```python
from build123d import *

# Parameters (mm, degrees)
SKETCH1_W       = 3
SKETCH1_H       = 12
SKETCH5_W       = 2.05
SKETCH5_H       = 0.74
CHANFREIN1_SIZE = 0.2


with BuildPart() as part:
    # Sketch1 → Revolve1 (revolve)
    with BuildSketch(Plane.XY):
        with Locations((1.5, 6)):
            Rectangle(SKETCH1_W, SKETCH1_H)
    revolve(axis=Axis((0, 0, 0), (0, 1, 0)))

    # Sketch5 → Groove for DIN 471 - 4 x 0.4, Circlip for shafts - normal1 (revolve, cut)
    with BuildSketch(Plane(origin=(0, 0, 0), x_dir=(0, 0, -1), z_dir=(-1, 0, 0))):
        with Locations((3.525, -10.97)):
            Rectangle(SKETCH5_W, SKETCH5_H)
    revolve(axis=Axis((0, 50.028808754, 0), (0, -1, 0)), mode=Mode.SUBTRACT)

    # Chanfrein1
    chanfrein1_edges = [part.edges().sort_by_distance(p)[0] for p in [
        (-3, 0, 0),
        (-3, 12, 0),
    ]]
    chamfer(chanfrein1_edges, length=CHANFREIN1_SIZE)


solid = part.part
```
Verification items for the finished model (mm, model axes). A direction names the side the tool comes from. Round coordinates to 2 decimals unless told otherwise and drop trailing zeros. Write each loop counter-clockwise with the first axis right and the second up, starting at its lowest first coordinate (ties: lowest second). Pieces come first, ordered by that corner, then holes. Notation, with made-up numbers: (84.25, 48.5) - (111.25, 48.5) arc R20 cw to (111.25, 63.5) - close; hole circle Ø4 at (68, 70). An arc over 180 degrees is marked (long way). Answer as a JSON object with one key per item and string values. Group by question number.
Q1. Section check A-A, the plane y = 11. Enter the section's corners in (x, z).
Q2. Section check B-B, the plane y = 5. Enter the section's corners in (x, z), plus the area to 3 significant figures.
Q3. Thickness scan on line 1 (Y direction, x = 0.9, z = -2.55); line 2 (Z direction, x = -1.7, y = 8.75); line 3 (Z direction, x = -1, y = 8.75). Record the ranges inside material, lowest first.
Q4. Go/stop test with a flat-tipped pin: pin 1 Ø3 at (x, y) = (2, 10.5) entering from -Z. Record where the tip stops, or that it passes through.
Q5. Tool access check on faces 1 (the cylindrical face through (-2.44, 10.96, 0.54)), 2 (the cylindrical face through (-3, 11.6, -0.1)). Record the directions out of +Z, -Z, +X, -X, +Y, -Y that give a thin tool (end or side, any length) a straight path to the whole face; none if there is none.
Q6. Mould release check, pull along Y, two halves, no side actions. Record for faces 3 (the flat face through (2, 11.34, -2)), 4 (the flat face through (0, 0, 0)), 5 (the flat face through (0, 12, 0)): released by +Y, released by -Y, zero draft, split by the parting line, or undercut.
Found:
{
 "1": {"outline": "circle Ø5 at (0, 0)"},
 "2": {"outline": "circle Ø6 at (0, 0)", "area": "28.3 mm^2"},
 "3": {"line 1": "y = 0 to 10.6, 11.34 to 12", "line 2": "z = -2.47 to 2.47", "line 3": "z = -2.83 to 2.83"},
 "4": {"pin 1": "stops at z = -2.96"},
 "5": {"face 1": "none", "face 2": "+Y, -Y"},
 "6": {"face 3": "undercut", "face 4": "released by -Y", "face 5": "released by +Y"}
}
